```python
from build123d import *

# Parameters (mm, degrees)
SKETCH_1_W          = 25
SKETCH_1_H          = 24
EXTRUDE_1_DEPTH     = 2
SKETCH_2_W          = 8.5
SKETCH_2_H          = 8.5
EXTRUDE_2_DEPTH     = 2
SKETCH_3_R          = 3.5
EXTRUDE_3_DEPTH     = 1
FILLET_1_R          = 3
FILLET_2_R          = 3
FILLET_3_R          = 3
FILLET_4_R          = 3
SKETCH_5_R          = 1.34400515
SKETCH_5_R_2        = 1.577179003
CUT_EXTRUDE_1_DEPTH = 21


with BuildPart() as part:
    # 스케치1 → 보스-돌출1 (new body)
    with BuildSketch(Plane.XY):
        Rectangle(SKETCH_1_W, SKETCH_1_H)
    extrude(amount=EXTRUDE_1_DEPTH)

    # 스케치2 → 보스-돌출2 (add)
    with BuildSketch(Plane.XY.offset(2)):
        with Locations((0, 2.55)):
            Rectangle(SKETCH_2_W, SKETCH_2_H)
    extrude(amount=EXTRUDE_2_DEPTH)

    # 스케치3 → 보스-돌출3 (add)
    with BuildSketch(Plane.XY.offset(4)):
        with Locations((0, 2.55)):
            Circle(SKETCH_3_R)
    extrude(amount=EXTRUDE_3_DEPTH)

    # 필렛1
    fillet_1_edges = [part.edges().sort_by_distance(p)[0] for p in [
        (-12.5, -12, 1),
    ]]
    fillet(fillet_1_edges, radius=FILLET_1_R)

    # 필렛2
    fillet_2_edges = [part.edges().sort_by_distance(p)[0] for p in [
        (-12.5, 12, 1),
    ]]
    fillet(fillet_2_edges, radius=FILLET_2_R)

    # 필렛3
    fillet_3_edges = [part.edges().sort_by_distance(p)[0] for p in [
        (12.5, 12, 1),
    ]]
    fillet(fillet_3_edges, radius=FILLET_3_R)

    # 필렛4
    fillet_4_edges = [part.edges().sort_by_distance(p)[0] for p in [
        (12.5, -12, 1),
    ]]
    fillet(fillet_4_edges, radius=FILLET_4_R)

    # 스케치5 → 컷-돌출1 (cut)
    with BuildSketch(Plane.XY.offset(2)):
        with Locations((-10.027820436, 2.115243373)):
            Circle(SKETCH_5_R)
        with Locations((10.027820436, 2.115243373)):
            Circle(SKETCH_5_R)
        with Locations((-9.5, -9)):
            Circle(SKETCH_5_R_2)
        with Locations((9.5, -9)):
            Circle(SKETCH_5_R_2)
    extrude(amount=-CUT_EXTRUDE_1_DEPTH, mode=Mode.SUBTRACT)


solid = part.part
```
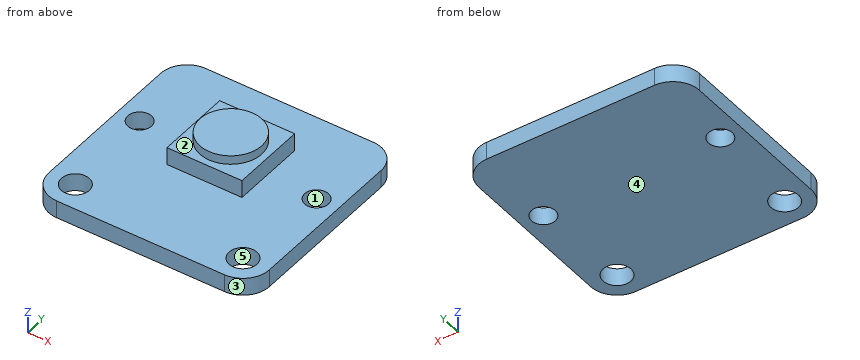
The listing builds one solid part. Answer for the finished solid, in the listing's coordinates (mm). Face numbers are marked on the shaded views. A direction names the side the tool comes from. Give positions to 0.01 mm unless a question says otherwise; leave off trailing zeros. Order: outer loops, then holes, each group sorted by start corner. A loop starts at its lowest first (then second) coordinate and runs counter-clockwise, first axis right, second up. Notation, with made-up numbers: (68.5, 9.5) -> (90.5, 9.5) arc R35 ccw to (90.5, 46.5) -> close; hole circle Ø8 at (-34.5, 78). An arc over 180 degrees is marked (long way). Answer as a JSON object with one key per item and string values. Group by question number.
Item 1: A tool of negligible diameter and unlimited length cuts with its end or side. For the marked faces 1 and 2, from which of +Z, -Z, +X, -X, +Y, -Y can it reach the whole face along a straight path? Write none if from no direction.
Item 2: The part is cut by section A-A on x = 0. Write down the section's boundary in (y, z).
Item 3: Flat-ended cylindrical pins translate along their axes: pin 1 (0.6 mm diameter, centred on x = -1, z = 3, fed in from +Y); pin 2 (3 mm diameter, centred on y = 3, z = 4, fed in from -X); pin 3 (4 mm diameter, centred on x = -7, y = 0, fed in from +Z). Find the tip coordinate at first contact, or state that the pin passes through.
Item 4: Consider L1, parallel to X at y = 1.75, z = 0.35; L2, parallel to Z at x = -1.75, y = 7; L3, parallel to X at y = 6.25, z = 3.85. Determine where each line is inside the solid, lowest interval first. Write a range as from..to.
Item 5: The part is cut by section B-B on y = 2.55. Write down the section's boundary in (x, z).
Item 6: The part is cut by section C-C on x = -10.75. Write down the section's boundary in (y, z), and give its area (3 significant figures).
Item 7: The part is cut by section D-D on z = 1.15. Write down the section's boundary in (x, y), and give its area (3 significant figures).
Item 8: Determine the mould class of the marked faces 3, 4 and 5 for opening direction X: pulls with the +X half, pulls with the -X half, needs draft (parallel to the pull), parting line crosses it, or undercut.
Result set:
{
 "1": {"face 1": "+Z, -Z", "face 2": "+Z"},
 "2": {"outline": "(-12, 0) -> (12, 0) -> (12, 2) -> (6.8, 2) -> (6.8, 4) -> (6.05, 4) -> (6.05, 5) -> (-0.95, 5) -> (-0.95, 4) -> (-1.7, 4) -> (-1.7, 2) -> (-12, 2) -> close"},
 "3": {"pin 1": "y = 6.8", "pin 2": "x = -4.25", "pin 3": "z = 2"},
 "4": {"L1": "-12.5..-11.32, -8.73..8.73, 11.32..12.5", "L2": "0..2", "L3": "-4.25..4.25"},
 "5": {"outline": "(-12.5, 0) -> (-11.3, 0) -> (-11.3, 2) -> (-12.5, 2) -> close; (-8.76, 0) -> (8.76, 0) -> (8.76, 2) -> (4.25, 2) -> (4.25, 4) -> (3.5, 4) -> (3.5, 5) -> (-3.5, 5) -> (-3.5, 4) -> (-4.25, 4) -> (-4.25, 2) -> (-8.76, 2) -> close; (11.3, 0) -> (12.5, 0) -> (12.5, 2) -> (11.3, 2) -> close"},
 "6": {"outline": "(-11.73, 0) -> (-9.96, 0) -> (-9.96, 2) -> (-11.73, 2) -> close; (-8.04, 0) -> (0.98, 0) -> (0.98, 2) -> (-8.04, 2) -> close; (3.25, 0) -> (11.73, 0) -> (11.73, 2) -> (3.25, 2) -> close", "area": "38.5 mm²"},
 "7": {"outline": "(-12.5, -9) arc R3 ccw to (-9.5, -12) -> (9.5, -12) arc R3 ccw to (12.5, -9) -> (12.5, 9) arc R3 ccw to (9.5, 12) -> (-9.5, 12) arc R3 ccw to (-12.5, 9) -> close; hole circle Ø2.69 at (-10.03, 2.12); hole circle Ø3.15 at (-9.5, -9); hole circle Ø3.15 at (9.5, -9); hole circle Ø2.69 at (10.03, 2.12)", "area": "565 mm²"},
 "8": {"face 3": "pulls with the +X half", "face 4": "needs draft", "face 5": "undercut"}
}
